Read the model definition and answer for the solid it produces. Units are mm, in the model's axes. Face numbers are marked on the shaded views. Round coordinates to 2 decimals unless told otherwise and drop trailing zeros. Order: outer loops, then holes, each group sorted by start corner. A loop starts at its lowest first (then second) coordinate and runs counter-clockwise, first axis right, second up. Notation, with made-up numbers: (-26.75, 85) - (1.25, 85) arc R22 cw to (1.25, 122) - close; hole circle Ø7 at (18.25, -38.75). An arc over 180 degrees is marked (long way). Answer as a JSON object with one key per item and string values. Group by question number.
Q1. The mould has two halves that part along Y. Classify the marked faces 1, 2 and 3: pulls with the +Y half, pulls with the -Y half, needs draft (parallel to the pull), parting line crosses it, or undercut.
Q2. A cutting plane is placed at A-A on z = -37. Determine the outline of the cut face in (x, y).
Q3. Consider line 1 (Y direction, x = 0, z = -24); line 2 (X direction, y = -0.5, z = -19.5). Determine where each line is inside the solid, lowest interval first.
Q4. A cutting plane is placed at B-B on z = -7. Determine the outline of the cut face in (x, y), and give its area (3 significant figures).
Q5. Given pin 1 Ø4 at (x, y) = (-5.5, 16.5) entering from +Z; pin 2 Ø4 at (x, y) = (-22, -24) entering from -Z; pin 3 Ø6 at (y, z) = (5.5, -20.5) entering from +X, each flat-ended and moving along its own axis, determine where each tip first touches the part or whether it passes through.
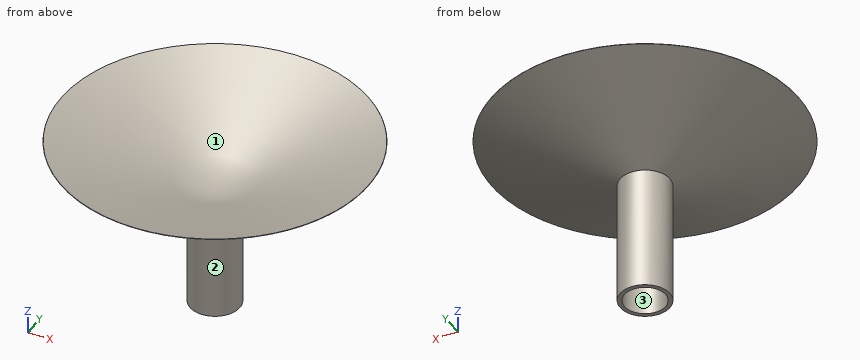
Autodesk Inventor part; units mm, degrees
ref_plane "YZ Plane" through (0, 0, 0) normal (1, 0, 0) x (0, 1, 0)
ref_plane "XZ Plane" through (0, 0, 0) normal (0, 1, 0) x (-1, 0, 0)
ref_plane "XY Plane" through (0, 0, 0) normal (0, 0, 1) x (1, 0, 0)
sketch "Sketch2" plane through (0, 0, 0) normal (0, 1, 0) x (-1, 0, 0)
  line L0 (37, 0) -> (0, -13.4669)
  line L1 (37, 0) -> (76.3746, 0) construction
  line L2 (0, -13.4669) -> (0, -13.5669)
  line L3 (0, -13.5669) -> (37.0321, -0.0883)
  line L4 (37.0321, -0.0883) -> (37, 0)
  line L5 (0, -16.2803) -> (0, 2.7134)
  point P0 (0, 0)
  dimension "d5" = 160
  dimension "d6" = 0.1
  dimension "d7" = 110
  dimension "d8" = 70
revolve "Revolution2" add sketch "Sketch2" angle 360 about axis through (0, 0, -10) along (0, 0, 1)
sketch "Sketch3" plane through (0, 0, 0) normal (0, 1, 0) x (-1, 0, 0)
  line L0 (-37, 0) -> (0, -13.4669)
  line L1 (-5, -11.647) -> (-5, -41.647)
  line L2 (-5, -41.647) -> (-6, -41.647)
  line L3 (-6, -41.647) -> (-6, -11.647)
  line L4 (-6, -11.647) -> (-5, -11.647)
  line L5 (0, -37.9765) -> (0, 6.3294)
  point P0 (0, 0)
  dimension "d10" = 30
  dimension "d11" = 1
  dimension "d12" = 90
  dimension "d13" = 30
  dimension "d14" = 90
revolve "Revolution3" add sketch "Sketch3" angle 360 about axis through (0, 0, -10) along (0, 0, 1)
properties part number "small_membrane"
Result set:
{
 "1": {"face 1": "undercut", "face 2": "parting line crosses it", "face 3": "undercut"},
 "2": {"outline": "circle Ø12 at (0, 0); hole circle Ø10 at (0, 0)"},
 "3": {"line 1": "y = -6 to -5, 5 to 6", "line 2": "x = -5.98 to -4.97, 4.97 to 5.98"},
 "4": {"outline": "circle Ø36.08 at (0, 0); hole circle Ø35.54 at (0, 0)", "area": "30.9 mm²"},
 "5": {"pin 1": "stops at z = -6.41", "pin 2": "stops at z = -2.44", "pin 3": "stops at x = 5.45"}
}
